from build123d import *
from build123d.topology import SkipClean

# Parameters (mm, degrees)
BASE_FLANGE1_DEPTH  = 102.87
CUT_EXTRUDE1_START  = -7.62
CUT_EXTRUDE1_DEPTH  = 7.62
BOSS_EXTRUDE5_START = -95.25
BOSS_EXTRUDE5_DEPTH = 95.25
BOSS_EXTRUDE6_DEPTH = 10.16
BOSS_EXTRUDE7_DEPTH = 0.762
SKETCH12_W          = 72.378245623
SKETCH12_H          = 0.762
BOSS_EXTRUDE8_DEPTH = 12.7
SKETCH13_R          = 3.175
CUT_EXTRUDE2_DEPTH  = 204.597121983
BOSS_EXTRUDE9_START = 3.81
BOSS_EXTRUDE9_DEPTH = 3.81


# Read off the part's stored shape, not the designer's step: Cut-Extrude1
# Sheet-metal steps are written as plain solids
with BuildPart() as part:
    # Sketch2 → Base-Flange1 (new body)
    with BuildSketch(Plane(origin=(0, 0, 0), x_dir=(1, 0, 0), z_dir=(0, 1, 0))):
        with BuildLine():
            ThreePointArc((-119.38, 0), (35.898258345, 113.85472958), (97.790371047, -68.473554972))
            Line((97.790371047, -68.473554972), (97.186983651, -68.051058569))
            ThreePointArc((97.186983651, -68.051058569), (35.676758453, 113.152221674), (-118.6434, 0))
            Line((-118.6434, 0), (-119.38, 0))
        make_face()
    extrude(amount=BASE_FLANGE1_DEPTH)

    # Cut-Extrude1 outline → Cut-Extrude1 (cut)
    with BuildSketch(Plane.XZ.offset(CUT_EXTRUDE1_START)):
        with BuildLine():
            ThreePointArc((-119.38, 0), (18.160489843, -117.990597119), (113.85472958, 35.898258345))
            Line((113.85472958, 35.898258345), (113.152221674, 35.676758453))
            ThreePointArc((113.152221674, 35.676758453), (18.048435757, -117.262570031), (-118.6434, 0))
            Line((-118.6434, 0), (-119.38, 0))
        make_face()
    extrude(amount=CUT_EXTRUDE1_DEPTH, mode=Mode.SUBTRACT)

    # Sketch9 → Boss-Extrude5 (add)
    with BuildSketch(Plane(origin=(0, 102.87, 0), x_dir=(1, 0, 0), z_dir=(0, 1, 0)).offset(BOSS_EXTRUDE5_START)):
        with BuildLine():
            Line((-119.379693576, -0.270484204), (-118.6434, 0))
            Line((-118.6434, 0), (-119.38, 0))
            ThreePointArc((-119.38, 0), (-119.379923394, -0.135242189), (-119.379693576, -0.270484204))
        make_face()
    extrude(amount=BOSS_EXTRUDE5_DEPTH)

    # Sketch10 → Boss-Extrude6 (add)
    with SkipClean():  # the faces are left unmerged after this step: merging them gives an invalid solid
        with BuildSketch(Plane(origin=(0, 102.87, 0), x_dir=(1, 0, 0), z_dir=(0, 1, 0))):
            with BuildLine():
                Line((-119.379693576, -0.270484204), (-118.6434, 0))
                ThreePointArc((-118.6434, 0), (-107.527437301, 50.140867475), (-76.262507491, 90.886117283))
                Line((-76.262507491, 90.886117283), (-76.735984844, 91.45038562))
                ThreePointArc((-76.735984844, 91.45038562), (-108.252110006, 50.329564663), (-119.379693576, -0.270484204))
            make_face()
        extrude(amount=BOSS_EXTRUDE6_DEPTH)

    # Sketch11 → Boss-Extrude7 (add)
    with SkipClean():  # the faces are left unmerged after this step: merging them gives an invalid solid
        with BuildSketch(Plane(origin=(0, 113.03, 0), x_dir=(1, 0, 0), z_dir=(0, 1, 0))):
            with BuildLine():
                Line((-119.379693576, -0.270484204), (-51.440692331, 24.687531528))
                Line((-51.440692331, 24.687531528), (-76.735984844, 91.45038562))
                ThreePointArc((-76.735984844, 91.45038562), (-108.252110006, 50.329564663), (-119.379693576, -0.270484204))
            make_face()
        extrude(amount=BOSS_EXTRUDE7_DEPTH)

    # Sketch12 → Boss-Extrude8 (add)
    with SkipClean():  # the faces are left unmerged after this step: merging them gives an invalid solid
        with BuildSketch(Plane(origin=(-14.107419738, 0, -38.402251904), x_dir=(0.9386660406079884, 0, -0.3448275862069655), z_dir=(0.3448275862069655, 0, 0.9386660406079884))):
            with Locations((-75.961811901, 113.411)):
                Rectangle(SKETCH12_W, SKETCH12_H)
        extrude(amount=BOSS_EXTRUDE8_DEPTH)

    # Sketch13 → Cut-Extrude2 (cut, through all)
    with SkipClean():  # the faces are left unmerged after this step: merging them gives an invalid solid
        with BuildSketch(Plane(origin=(0, 113.792, 0), x_dir=(1, 0, 0), z_dir=(0, 1, 0))):
            with Locations(Location((-94.540026844, 2.089676094, 0), (0, 0, 270))):
                Circle(SKETCH13_R)
            with Locations(Location((-71.890015284, 10.410365749, 0), (0, 0, 270))):
                Circle(SKETCH13_R)
        extrude(amount=-CUT_EXTRUDE2_DEPTH, mode=Mode.SUBTRACT)

    # Sketch14 → Boss-Extrude9 (add)
    with SkipClean():  # the faces are left unmerged after this step: merging them gives an invalid solid
        with BuildSketch(Plane.XZ.offset(BOSS_EXTRUDE9_START)):
            with BuildLine():
                Line((97.186983651, 68.051058569), (119.774310511, 76.632245246))
                ThreePointArc((119.774310511, 76.632245246), (130.778139327, 73.589906503), (131.18256886, 62.180414385))
                Line((131.18256886, 62.180414385), (113.152221674, 35.676758453))
                ThreePointArc((113.152221674, 35.676758453), (106.408031423, 52.474633989), (97.186983651, 68.051058569))
            make_face()
            with BuildLine():
                ThreePointArc((126.590987662, 68.955600398), (122.972686098, 71.90312373), (120.025162766, 68.284822166))
                ThreePointArc((120.025162766, 68.284822166), (123.64346433, 65.337298834), (126.590987662, 68.955600398))
            make_face(mode=Mode.SUBTRACT)
        extrude(amount=-BOSS_EXTRUDE9_DEPTH)


solid = part.part
Read the model definition and answer for the solid it produces. Units are mm, in the model's axes. A direction names the side the tool comes from. Give positions to 0.01 mm unless a question says otherwise; leave off trailing zeros. Write each loop counter-clockwise with the first axis right and the second up, starting at its lowest first coordinate (ties: lowest second). Pieces come first, ordered by that corner, then holes. Notation, with made-up numbers: (-2.5, 30.25) -> (10.5, 30.25) arc R21 ccw to (10.5, 46.25) -> close; hole circle Ø3 at (84, -6.75). An arc over 180 degrees is marked (long way). Answer as a JSON object with one key per item and string values. Group by question number.
1) Find section D-D (z = -77). Write down the section's boundary in (x, y), and give its area (3 significant figures).
2) Find section B-B (y = 66). Write down the section's boundary in (x, z), and give its area (3 significant figures).
3) Each of these flat-tipped pins is pushed along its axis until it touches: P1, Ø5, axis at x = -71.89, z = -10.41, coming from the +Y side; P2, Ø8, axis at x = -38.5, y = 26, coming from the -Z side; P3, Ø8.5, axis at x = 123.31, z = 68.62, coming from the +Y side; P4, Ø5, axis at y = 13, z = 21, coming from the +X side. Where does it stop, or does it pass through?
4) A tool of negligible diameter and unlimited length cuts with its end or side. For faces 1 (the flat face through (115, -3.81, 61)), 2 (the flat face through (116, 0, 62)), from which of +Z, -Z, +X, -X, +Y, -Y can it reach the whole face along a straight path? Write none if from no direction.
5) Consider L1, parallel to X at y = 71.5, z = -55.5; L2, parallel to Z at x = 109.5, y = 13.5; L3, parallel to Y at x = -59, z = -8.5. Determine where each line is inside the solid, lowest interval first. Write a range as from..to.
6) The mould has two halves that part along X. Classify faces 3 (the cylindrical face through (120.28, -1.93, 67.31)), 4 (the flat face through (122.29, -1.93, 49.11)), 5 (the flat face through (-84, 113.03, -29)): +X half, -X half, draft (parallel to the pull), parting line (faces both ways), or undercut.
7) Find section A-A (z = -35). Write down the section's boundary in (x, y).
Values follow:
{
 "1": {"outline": "(-91.23, 7.62) -> (-90.26, 7.62) -> (-90.26, 113.03) -> (-71.26, 113.03) -> (-71.26, 113.79) -> (-91.23, 113.79) -> close; (90.26, 7.62) -> (91.23, 7.62) -> (91.23, 102.87) -> (90.26, 102.87) -> close", "area": "209 mm2"},
 "2": {"outline": "(-119.38, 0) arc R119.38 ccw (long way) to (97.79, 68.47) -> (97.19, 68.05) arc R118.64 cw (long way) to (-118.64, 0) -> (-119.38, 0.27) arc R119.38 ccw to start", "area": "329 mm2"},
 "3": {"P1": "passes through", "P2": "stops at z = -114.29", "P3": "stops at y = 0", "P4": "stops at x = 117.94"},
 "4": {"face 1": "+Z, -Z, +X, -X, -Y", "face 2": "+Z, +X, +Y"},
 "5": {"L1": "x = -105.69..-104.86, 104.86..105.69", "L2": "z = -47.55..-45.67, 45.67..47.55", "L3": "y = 113.03..113.79"},
 "6": {"face 3": "undercut", "face 4": "+X half", "face 5": "draft"},
 "7": {"outline": "(-114.13, 7.62) -> (-113.36, 7.62) -> (-113.36, 113.03) -> (-55.35, 113.03) -> (-55.35, 113.79) -> (-114.13, 113.79) -> close; (113.36, 7.62) -> (114.13, 7.62) -> (114.13, 102.87) -> (113.36, 102.87) -> close"}
}
